from build123d import *

# Parameters (mm, degrees)
F1_DEPTH = 400
F2_T     = -1


with BuildPart() as f1:
    # F0 (on Front) → F1 (new body)
    with BuildSketch(Plane.XZ):
        Polygon((0, 400), (0, 0), (400, 0), (1600, 600), (2000, 600), (2000, 1000), (1600, 1000), (400, 400), align=None)
    extrude(amount=F1_DEPTH)

    # F2
    f2_openings = [f1.faces().sort_by_distance(p)[0] for p in [
        (200, -200, 400),
        (1000, -200, 700),
        (1800, -200, 1000),
    ]]
    offset(amount=F2_T, openings=f2_openings, kind=Kind.INTERSECTION)


solid = f1.part
Read the model definition and answer for the solid it produces. Units are mm, in the model's axes. A direction names the side the tool comes from. Give positions to 0.01 mm unless a question says otherwise; leave off trailing zeros. Write each loop counter-clockwise with the first axis right and the second up, starting at its lowest first coordinate (ties: lowest second). Pieces come first, ordered by that corner, then holes. Notation, with made-up numbers: (74.5, -24.5) -> (118.5, -24.5) arc R19 ccw to (118.5, 10.5) -> close; hole circle Ø1 at (83.5, -30). An arc over 180 degrees is marked (long way). Answer as a JSON object with one key per item and string values. Group by question number.
1) A tool of negligible diameter and unlimited length cuts with its end or side. For faces 1 (the flat face through (1999, -197, 798)), 2 (the flat face through (197, -197, 0)), 3 (the flat face through (986, -399, 507)), 4 (the flat face through (1797, -197, 600)), 5 (the flat face through (1008.4, -399.5, 704.2)), from which of +Z, -Z, +X, -X, +Y, -Y can it reach the whole face along a straight path? Write none if from no direction.
2) The mould has two halves that part along X. Classify faces 6 (the flat face through (0, -197, 203)), 7 (the flat face through (1797, -197, 601)), 8 (the flat face through (986, -1, 507)): +X half, -X half, draft (parallel to the pull), parting line (faces both ways), or undercut.
3) Consider L1, parallel to Y at x = 750, z = 250; L2, parallel to X at y = -36, z = 842; L3, parallel to X at y = -33.5, z = 213.5. Determine where each line is inside the solid, lowest interval first. Write a range as from..to.
4) Find section C-C (z = 214.5). Write down the section's boundary in (x, y).
5) Find section D-D (x = 1262.5). Write down the section's boundary in (y, z).
6) Find section B-B (y = -322.5). Write down the section's boundary in (x, z), and give its area (3 significant figures).
7) Find section A-A (z = 643.5). Write down the section's boundary in (x, y), and give its area (3 significant figures).
8) Each of these flat-tipped pins is pushed along its axis until it touches: P1, Ø10, axis at x = 977.5, y = -327.5, coming from the +Z side; P2, Ø12, axis at x = 1509.5, y = -104.5, coming from the +Z side; P3, Ø3, axis at x = 671.5, z = 322.5, coming from the +Y side; P4, Ø6, axis at x = 1173, y = -239.5, coming from the +Z side. Where does it stop, or does it pass through?
Values follow:
{
 "1": {"face 1": "+Z, -X", "face 2": "-Z, +X, -X, +Y, -Y", "face 3": "+Z", "face 4": "-Z, +X, +Y, -Y", "face 5": "+Z, -X, +Y, -Y"},
 "2": {"face 6": "-X half", "face 7": "draft", "face 8": "undercut"},
 "3": {"L1": "y = -400..-399, -1..0", "L2": "x = 1999..2000", "L3": "x = 0..1, 824.76..827"},
 "4": {"outline": "(0, -400) -> (829, -400) -> (829, 0) -> (0, 0) -> close; hole (1, -399) -> (826.76, -399) -> (826.76, -1) -> (1, -1) -> close"},
 "5": {"outline": "(-400, 431.25) -> (0, 431.25) -> (0, 831.25) -> (-1, 831.25) -> (-1, 432.37) -> (-399, 432.37) -> (-399, 831.25) -> (-400, 831.25) -> close"},
 "6": {"outline": "(0, 0) -> (400, 0) -> (1600, 600) -> (2000, 600) -> (2000, 1000) -> (1999, 1000) -> (1999, 601) -> (1599.76, 601) -> (399.76, 1) -> (1, 1) -> (1, 400) -> (0, 400) -> close", "area": "2,940 mm2"},
 "7": {"outline": "(887, -400) -> (2000, -400) -> (2000, 0) -> (887, 0) -> (887, -1) -> (1999, -1) -> (1999, -399) -> (887, -399) -> close", "area": "2,620 mm2"},
 "8": {"P1": "stops at z = 292.37", "P2": "stops at z = 558.87", "P3": "stops at y = 0", "P4": "stops at z = 389.12"}
}
